Input: part model. Units: mm. Frame: model coordinates. A direction names the side the tool comes from. Round coordinates to 2 decimals unless told otherwise and drop trailing zeros. Loops run counter-clockwise (first coordinate to the right, second up) from the corner with the lowest first, then second, coordinate; pieces in that order, holes last. Notation, with made-up numbers: (70.25, 64) -> (107.25, 64) arc R7 cw to (107.25, 75) -> close; hole circle Ø8 at (76, -38). An arc over 180 degrees is marked (long way). Answer as a JSON object with one key per item and string values. Group by question number.
Item 1: Draft query along X for faces 5 (the flat face through (45, 7, -40)), 6 (the flat face through (24, 7, 50)), 7 (the flat face through (-41.372, 6.916, 24.65)). Return one class per face: released by +X, released by -X, zero draft, split by the parting line, or undercut.
Item 2: Section query C-C on y = 7.25. Return loops of the section in (x, z).
Item 3: Section query B-B on z = 13. Return loops of the section in (x, y), and give its area (3 significant figures).
Item 4: Pin query (flat end, axial travel): pin 1 (7 mm diameter, centred on x = 22.5, y = 5, fed in from -Z); pin 2 (7 mm diameter, centred on y = 5, z = 40.5, fed in from -X); pin 3 (6 mm diameter, centred on y = 3.5, z = 40, fed in from +X). Return the tip coordinate at first contact, or that it passes through.
Item 5: Set-up query: faces 1 (the flat face through (-15, 7, 40)), 2 (the flat face through (15, 12, 40)), 3 (the flat face through (15, 7, -40)), 4 (the flat face through (48, 7, -50)). Return all of +Z, -Z, +X, -X, +Y, -Y with unobstructed straight access to the full face (end or side cutting, diameter ignored); none if empty.
Item 6: Material intervals for line 1 (X direction, y = 10, z = -44); line 2 (Z direction, x = -30, y = 8.75); line 3 (Z direction, x = -6.5, y = 12.75), sorted ascending. Write a range as [from, to].
Item 7: Section query A-A on z = -41. Return loops of the section in (x, y), and give its area (3 significant figures).
Item 8: Section query D-D on x = 2. Return loops of the section in (y, z).
from build123d import *

# Parameters (mm, degrees)
BOSS_EXTRUDE1_DEPTH = 14.027771651
CUT_EXTRUDE1_DEPTH  = 16
CUT_EXTRUDE2_DEPTH  = 16


with BuildPart() as part:
    # Sketch1 → Boss-Extrude1 (new body)
    with BuildSketch(Plane(origin=(0, 0, 0), x_dir=(1, 0, 0), z_dir=(0, 1, 0))):
        Polygon((-45, 50), (-50, 50), (-50, -50), (-15, -50), (-15, -30), (15, -30), (15, -50), (50, -50), (50, 50), (45, 50), (45, 30), (15, 30), (15, 50), (-15, 50), (-15, 30), (-45, 30), align=None)
    extrude(amount=BOSS_EXTRUDE1_DEPTH)

    # Sketch2 → Revolve1 (revolve)
    with BuildSketch(Plane.ZY.offset(-15)):
        with BuildLine():
            Line((40.205231865, 11.565079329), (40.205231865, 1.565079329))
            ThreePointArc((40.205231865, 1.565079329), (35.205231865, 6.565079329), (40.205231865, 11.565079329))
        make_face()
    revolve(axis=Axis((15, 11.565079329, 40.205231865), (0, -1, 0)))

    # Sketch3 → Cut-Extrude1 (cut)
    with BuildSketch(Plane(origin=(0, 0, 0), x_dir=(1, 0, 0), z_dir=(0, 1, 0))):
        Polygon((-50, 0), (-32.5, -50), (-50, -50), align=None)
    extrude(amount=CUT_EXTRUDE1_DEPTH, mode=Mode.SUBTRACT)

    # Sketch4 → Cut-Extrude2 (cut)
    with BuildSketch(Plane(origin=(0, 0, 0), x_dir=(1, 0, 0), z_dir=(0, 1, 0))):
        Polygon((32.5, -50), (50, 0), (50, -50), align=None)
    extrude(amount=CUT_EXTRUDE2_DEPTH, mode=Mode.SUBTRACT)


solid = part.part
Solved:
{
 "1": {"face 5": "undercut", "face 6": "zero draft", "face 7": "released by -X"},
 "2": {"outline": "(-50, -50) -> (-45, -50) -> (-45, -30) -> (-15, -30) -> (-15, -50) -> (15, -50) -> (15, -30) -> (45, -30) -> (45, -50) -> (50, -50) -> (50, 0) -> (32.5, 50) -> (15, 50) -> (15, 45.16) arc R4.95 ccw to (15, 35.25) -> (15, 30) -> (-15, 30) -> (-15, 50) -> (-32.5, 50) -> (-50, 0) -> close"},
 "3": {"outline": "(-45.45, 0) -> (45.45, 0) -> (45.45, 14.03) -> (-45.45, 14.03) -> close", "area": "1,280 mm²"},
 "4": {"pin 1": "z = -30", "pin 2": "x = -37.05", "pin 3": "x = 37.05"},
 "5": {"face 1": "+Z, +Y, -Y", "face 2": "none", "face 3": "-Z, +Y, -Y", "face 4": "-Z, +X, -X, +Y, -Y"},
 "6": {"line 1": "[-50, -45], [-15, 15], [45, 50]", "line 2": "[-30, 50]", "line 3": "[-50, 30]"},
 "7": {"outline": "(-50, 0) -> (-45, 0) -> (-45, 14.03) -> (-50, 14.03) -> close; (-15, 0) -> (15, 0) -> (15, 14.03) -> (-15, 14.03) -> close; (45, 0) -> (50, 0) -> (50, 14.03) -> (45, 14.03) -> close", "area": "561 mm²"},
 "8": {"outline": "(0, -50) -> (14.03, -50) -> (14.03, 30) -> (0, 30) -> close"}
}
